```python
from build123d import *

# Parameters (mm, degrees)
SKETCH1_R           = 7
BOSS_EXTRUDE1_DEPTH = 10
SKETCH2_R           = 56
BOSS_EXTRUDE2_DEPTH = 20
SKETCH3_R           = 3
SKETCH4_R           = 7.5
BOSS_EXTRUDE3_DEPTH = 25
CHAMFER1_SIZE       = 1
SKETCH5_R           = 45
CUT_EXTRUDE1_DEPTH  = 2
SCALE1_SCALE        = 0.18
SCALE2_SCALE        = 1.04


with BuildPart() as part:
    # Sketch1 → Boss-Extrude1 (new body)
    with BuildSketch(Plane(origin=(0, 0, 0), x_dir=(1, 0, 0), z_dir=(0, 1, 0))):
        with BuildLine():
            Line((-70.5, -70), (70.5, -70))
            ThreePointArc((70.5, -70), (82.52081528, -65.02081528), (87.5, -53))
            Line((87.5, -53), (87.5, 53))
            ThreePointArc((87.5, 53), (82.52081528, 65.02081528), (70.5, 70))
            Line((70.5, 70), (-70.5, 70))
            ThreePointArc((-70.5, 70), (-82.52081528, 65.02081528), (-87.5, 53))
            Line((-87.5, 53), (-87.5, -53))
            ThreePointArc((-87.5, -53), (-82.52081528, -65.02081528), (-70.5, -70))
        make_face()
        with Locations((-70.5, 53)):
            Circle(SKETCH1_R, mode=Mode.SUBTRACT)
        with Locations((-70.5, -53)):
            Circle(SKETCH1_R, mode=Mode.SUBTRACT)
        with Locations((70.5, -53)):
            Circle(SKETCH1_R, mode=Mode.SUBTRACT)
        with Locations((70.5, 53)):
            Circle(SKETCH1_R, mode=Mode.SUBTRACT)
    extrude(amount=BOSS_EXTRUDE1_DEPTH)

    # Sketch2 → Boss-Extrude2 (add)
    with BuildSketch(Plane.XZ):
        Circle(SKETCH2_R)
    extrude(amount=BOSS_EXTRUDE2_DEPTH)

    # Sketch3 → Revolve1 (revolve)
    with BuildSketch(Plane(origin=(0, 0, 0), x_dir=(0, 0, -1), z_dir=(1, 0, 0))):
        with Locations((-56, -17)):
            Circle(SKETCH3_R)
    revolve(axis=Axis((0, 0, 0), (0, -1, 0)))

    # Sketch4 → Boss-Extrude3 (add)
    with BuildSketch(Plane.XZ.offset(20)):
        Circle(SKETCH4_R)
    extrude(amount=BOSS_EXTRUDE3_DEPTH)

    # Chamfer1
    chamfer1_edges = [part.edges().sort_by_distance(p)[0] for p in [
        (-7.5, -45, 0),
    ]]
    chamfer(chamfer1_edges, length=CHAMFER1_SIZE)

    # Sketch5 → Cut-Extrude1 (cut)
    with BuildSketch(Plane(origin=(0, 10, 0), x_dir=(1, 0, 0), z_dir=(0, 1, 0))):
        Circle(SKETCH5_R)
    extrude(amount=-CUT_EXTRUDE1_DEPTH, mode=Mode.SUBTRACT)


with BuildPart() as part_1:
    # Scale1: scaled about (0, -2.631964086, 0)
    add(part.part.scale(SCALE1_SCALE).moved(Location((0, -2.158210551, 0))))


with BuildPart() as part_2:
    # Scale2: scaled about (0, -2.631964086, 0)
    add(part_1.part.scale(SCALE2_SCALE).moved(Location((0, 0.105278563, 0))))


solid = part_2.part
```
Geometry check sheet. Reference: the model listing, model coordinates, mm. A direction names the side the tool comes from. Give positions to 0.01 mm unless a question says otherwise; leave off trailing zeros. Order: outer loops, then holes, each group sorted by start corner. A loop starts at its lowest first (then second) coordinate and runs counter-clockwise, first axis right, second up. Notation, with made-up numbers: (36.25, 47) -> (53.25, 47) arc R16 ccw to (53.25, 53) -> close; hole circle Ø3 at (-22, -2.75). An arc over 180 degrees is marked (long way). Write each question's results on one line, items separated by ' | '. Start each with the question number.
(1) Sectioned sample at C-C (z = 0). Enter the section's corners in (x, y).
(2) Sectioned sample at A-A (y = -1.75). Enter the section's corners in (x, z), plus the area to 3 significant figures.
(3) Sectioned sample at B-B (x = 0). Enter the section's corners in (y, z), plus the area to 3 significant figures.
(4) Scan lines: line 1 (Y direction, x = 7.5, z = 5.5); line 2 (Y direction, x = -6, z = -11); line 3 (Z direction, x = 0, y = -0.5). Record each from-to range of solid material in increasing order.
(5) Access from +Z, -Z, +X, -X, +Y, -Y to the whole of each face (thin tool, end or side, straight path). Record for faces 1 (the face through (-1.4, -8.1, 0.1)), 2 (the face through (-15.42, -1.22, -12.2)), 3 (the face through (0, -0.642, 0)).
(6) Mould release check, pull along Y, two halves, no side actions. Record for faces 4 (the face through (-15.47, -1.22, 12.15)), 5 (the face through (-7.727, -3.431, 7.085)), 6 (the face through (0, -0.267, -9)): pulls with the +Y half, pulls with the -Y half, needs draft (parallel to the pull), parting line crosses it, or undercut.
(7) Sectioned sample at D-D (y = -4.25). Enter the section's corners in (x, z).
(8) Gauge pin test, flat ends, axial feed: P1, Ø1.5, axis at y = -4.5, z = 9, coming from the +X side (3 decimals); P2, Ø5, axis at y = -7.5, z = 7.5, coming from the +X side; P3, Ø4, axis at y = -6.5, z = -3, coming from the +X side. Record the tip position at first contact, or that the pin passes through.
Answer below:
1) outline: (-16.38, -2.14) -> (-10.48, -2.14) -> (-10.48, -4.76) arc R0.56 ccw to (-10.48, -5.88) -> (-1.4, -5.88) -> (-1.4, -10.38) -> (-1.22, -10.56) -> (1.22, -10.56) -> (1.4, -10.38) -> (1.4, -5.88) -> (10.48, -5.88) arc R0.56 ccw to (10.48, -4.76) -> (10.48, -2.14) -> (16.38, -2.14) -> (16.38, -0.27) -> (8.42, -0.27) -> (8.42, -0.64) -> (-8.42, -0.64) -> (-8.42, -0.27) -> (-16.38, -0.27) -> close
2) outline: (-16.38, -9.92) arc R3.18 ccw to (-13.2, -13.1) -> (13.2, -13.1) arc R3.18 ccw to (16.38, -9.92) -> (16.38, 9.92) arc R3.18 ccw to (13.2, 13.1) -> (-13.2, 13.1) arc R3.18 ccw to (-16.38, 9.92) -> close; hole circle Ø2.62 at (-13.2, -9.92); hole circle Ø2.62 at (-13.2, 9.92); hole circle Ø2.62 at (13.2, -9.92); hole circle Ø2.62 at (13.2, 9.92) | area: 828 mm2
3) outline: (-10.56, -1.22) -> (-10.38, -1.4) -> (-5.88, -1.4) -> (-5.88, -10.48) arc R0.56 ccw to (-4.76, -10.48) -> (-2.14, -10.48) -> (-2.14, -13.1) -> (-0.27, -13.1) -> (-0.27, -8.42) -> (-0.64, -8.42) -> (-0.64, 8.42) -> (-0.27, 8.42) -> (-0.27, 13.1) -> (-2.14, 13.1) -> (-2.14, 10.48) -> (-4.76, 10.48) arc R0.56 ccw to (-5.88, 10.48) -> (-5.88, 1.4) -> (-10.38, 1.4) -> (-10.56, 1.22) -> close | area: 135 mm2
4) line 1: -5.88 to -0.27 | line 2: -2.14 to -0.27 | line 3: -13.1 to -8.42, 8.42 to 13.1
5) face 1: -Y | face 2: -Z, -X, +Y, -Y | face 3: +Y
6) face 4: needs draft | face 5: undercut | face 6: pulls with the +Y half
7) outline: circle Ø20.97 at (0, 0)
8) P1: x = 6.965 | P2: x = 9.27 | P3: x = 10.96
